Geometry check sheet. Reference: the model listing, model coordinates, mm. Face numbers are marked on the shaded views. A direction names the side the tool comes from. Round coordinates to 2 decimals unless told otherwise and drop trailing zeros. Write each loop counter-clockwise with the first axis right and the second up, starting at its lowest first coordinate (ties: lowest second). Pieces come first, ordered by that corner, then holes. Notation, with made-up numbers: (64, 23) -> (114, 23) arc R25 ccw to (114, 48) -> close; hole circle Ø8 at (13.5, 55). An arc over 180 degrees is marked (long way). Use a Markdown table: item, result.
```python
from build123d import *

# Parameters (mm, degrees)
PAD_DEPTH    = 6
SKETCH002_W  = 39
SKETCH002_H  = 4
PAD001_DEPTH = 9
POCKET_DEPTH = 0.4


with BuildPart() as part:
    # Sketch001 → Pad (new body)
    with BuildSketch(Plane.XY):
        with BuildLine():
            Line((67.5, 0), (231.5, 0))
            Line((274, 42.5), (231.5, 0))
            Line((299, 42.5), (274, 42.5))
            Line((299, 42.5), (299, 67.5))
            Line((299, 67.5), (225, 67.5))
            ThreePointArc((225, 67.5), (223.585786, 66.914214), (223, 65.5))
            Line((223, 65.5), (223, 28.5))
            ThreePointArc((219.5, 25), (221.974874, 26.025126), (223, 28.5))
            Line((219.5, 25), (79.5, 25))
            ThreePointArc((76, 28.5), (77.025126, 26.025126), (79.5, 25))
            Line((76, 28.5), (76, 65.5))
            ThreePointArc((76, 65.5), (75.414214, 66.914214), (74, 67.5))
            Line((0, 67.5), (74, 67.5))
            Line((0, 67.5), (0, 42.5))
            Line((0, 42.5), (25, 42.5))
            Line((25, 42.5), (67.5, 0))
        make_face()
    extrude(amount=PAD_DEPTH)

    # Sketch002 → Pad001 (join)
    with BuildSketch(Plane.XY):
        with Locations((19.5, 69.5)):
            Rectangle(SKETCH002_W, SKETCH002_H)
        with Locations((279.5, 69.5)):
            Rectangle(SKETCH002_W, SKETCH002_H)
    extrude(amount=PAD001_DEPTH)

    # Sketch (on Face4 of Pad001) → Pocket (cut)
    with BuildSketch(Plane.XY.offset(6)):
        Polygon((144.9, 15.5), (149.5, 21.5), (154.1, 15.5), (150.9, 15.5), (150.9, 5.5), (148.1, 5.5), (148.1, 15.5), align=None)
        with BuildLine():
            ThreePointArc((168.193989, 19.692173), (156.5, 12.596087), (168.193989, 5.5))
            Line((167.122475, 8.086863), (168.193989, 5.5))
            ThreePointArc((167.122475, 17.105311), (159.283634, 12.596087), (167.122475, 8.086863))
            Line((167.122475, 17.105311), (168.193989, 19.692173))
        make_face()
    extrude(amount=-POCKET_DEPTH, mode=Mode.SUBTRACT)


solid = part.part
```
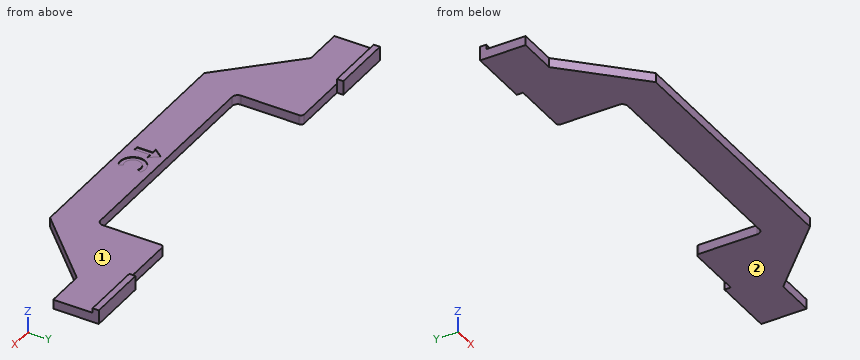
(1) Section check C-C on y = 35.5. Record the cut outline in (x, z).
A:
| item | result |
|---|---|
| outline | (32, 0) -> (76, 0) -> (76, 6) -> (32, 6) -> close; (223, 0) -> (267, 0) -> (267, 6) -> (223, 6) -> close |
(2) Gauge pin test, flat ends, axial feed: pin 1 Ø2 at (y, z) = (22.5, 5) entering from -X; pin 2 Ø1.5 at (x, z) = (26, 8) entering from -Y; pin 3 Ø4 at (x, z) = (251.5, 7) entering from -Y. Record the tip position at first contact, or that the pin passes through.
A:
| item | result |
|---|---|
| pin 1 | stops at x = 44 |
| pin 2 | stops at y = 67.5 |
| pin 3 | stops at y = 18.27 |
(3) Thickness scan on line 1 (Y direction, x = 164.5, z = 5.75); line 2 (X direction, y = 61.5, z = 4.5); line 3 (Z direction, x = 163, y = 24). Record the ranges inside material, lowest first.
A:
| item | result |
|---|---|
| line 1 | y = 0 to 4.6, 7.38 to 17.81, 20.6 to 25 |
| line 2 | x = 0 to 76, 223 to 299 |
| line 3 | z = 0 to 6 |
(4) Section check B-B on x = 164.5. Record the cut outline in (y, z), plus the area to 3 significant figures.
A:
| item | result |
|---|---|
| outline | (0, 0) -> (25, 0) -> (25, 6) -> (20.6, 6) -> (20.6, 5.6) -> (17.81, 5.6) -> (17.81, 6) -> (7.38, 6) -> (7.38, 5.6) -> (4.6, 5.6) -> (4.6, 6) -> (0, 6) -> close |
| area | 148 mm2 |
(5) Access from +Z, -Z, +X, -X, +Y, -Y to the whole of each face (thin tool, end or side, straight path). Record for the marked faces 1 and 2.
A:
| item | result |
|---|---|
| face 1 | +Z, +X, -X, -Y |
| face 2 | -Z, +X, -X, +Y, -Y |
(6) Section check A-A on y = 49.5. Record the cut outline in (x, z).
A:
| item | result |
|---|---|
| outline | (0, 0) -> (76, 0) -> (76, 6) -> (0, 6) -> close; (223, 0) -> (299, 0) -> (299, 6) -> (223, 6) -> close |
(7) Section check D-D on z = 4. Record the cut outline in (x, y).
A:
| item | result |
|---|---|
| outline | (0, 42.5) -> (25, 42.5) -> (67.5, 0) -> (231.5, 0) -> (274, 42.5) -> (299, 42.5) -> (299, 71.5) -> (260, 71.5) -> (260, 67.5) -> (225, 67.5) arc R2 ccw to (223, 65.5) -> (223, 28.5) arc R3.5 cw to (219.5, 25) -> (79.5, 25) arc R3.5 cw to (76, 28.5) -> (76, 65.5) arc R2 ccw to (74, 67.5) -> (39, 67.5) -> (39, 71.5) -> (0, 71.5) -> close |
